from build123d import *

# Parameters (mm, degrees)
BOSS_EXTRUDE1_DEPTH        = 120
BOSS_EXTRUDE2_DEPTH        = 20
CUT_EXTRUDE1_DEPTH         = 20
SKETCH17_W                 = 82.2
SKETCH17_H                 = 120
BOSS_EXTRUDE3_DEPTH        = 20
SKETCH18_W                 = 15.5
SKETCH18_H                 = 23
CUT_EXTRUDE2_DEPTH         = 20
SKETCH19_W                 = 15.5
SKETCH19_H                 = 23
BOSS_EXTRUDE4_DEPTH        = 20
CUT_EXTRUDE3_DEPTH         = 37
FILLET3_R                  = 3
SKETCH22_W                 = 30
SKETCH22_H                 = 120
BOSS_EXTRUDE5_DEPTH        = 5
SKETCH23_W                 = 30
SKETCH23_H                 = 120
BOSS_EXTRUDE6_DEPTH        = 5
F_8_CLEARANCE_HOLE1_REACH  = 187.624
F_8_CLEARANCE_HOLE1_BORE_R = 2.2479


with BuildPart() as part:
    # Sketch1 → Boss-Extrude1 (new body)
    with BuildSketch(Plane(origin=(0, 0, 0), x_dir=(1, 0, 0), z_dir=(0, 1, 0))):
        Polygon((-70, 15), (-70, -15), (70, -15), (70, 15), (60.3, 15), (60.3, -5), (50.8, -5), (50.8, 15), (41.1, 15), (41.1, -5), (-41.1, -5), (-41.1, 15), (-50.8, 15), (-50.8, -5), (-60.3, -5), (-60.3, 15), align=None)
    extrude(amount=BOSS_EXTRUDE1_DEPTH)

    # Sketch2 → Boss-Extrude2 (add)
    with BuildSketch(Plane(origin=(0, 120, 0), x_dir=(1, 0, 0), z_dir=(0, 1, 0))):
        Polygon((-63.3, -8), (-63.3, 15), (-60.3, 15), (-60.3, -5), (-50.8, -5), (-50.8, 15), (-47.8, 15), (-47.8, -8), align=None)
        Polygon((63.3, -8), (63.3, 15), (60.3, 15), (60.3, -5), (50.8, -5), (50.8, 15), (47.8, 15), (47.8, -8), align=None)
    extrude(amount=BOSS_EXTRUDE2_DEPTH)

    # Sketch3 → Cut-Extrude1 (cut)
    with BuildSketch(Plane.XZ):
        Polygon((-47.8, 8), (-47.8, -15), (-50.8, -15), (-50.8, 5), (-60.3, 5), (-60.3, -15), (-63.3, -15), (-63.3, 8), align=None)
        Polygon((63.3, 8), (63.3, -15), (60.3, -15), (60.3, 5), (50.8, 5), (50.8, -15), (47.8, -15), (47.8, 8), align=None)
    extrude(amount=-CUT_EXTRUDE1_DEPTH, mode=Mode.SUBTRACT)

    # Sketch17 → Boss-Extrude3 (add)
    with BuildSketch(Plane(origin=(0, 0, 5), x_dir=(-1, 0, 0), z_dir=(0, 0, -1))):
        with Locations((0, 60)):
            Rectangle(SKETCH17_W, SKETCH17_H)
    extrude(amount=BOSS_EXTRUDE3_DEPTH)

    # Sketch18 → Cut-Extrude2 (cut)
    with BuildSketch(Plane.XZ):
        with Locations((-25.05, -3.5)):
            Rectangle(SKETCH18_W, SKETCH18_H)
        with Locations((25.05, -3.5)):
            Rectangle(SKETCH18_W, SKETCH18_H)
    extrude(amount=-CUT_EXTRUDE2_DEPTH, mode=Mode.SUBTRACT)

    # Sketch19 → Boss-Extrude4 (add)
    with BuildSketch(Plane(origin=(0, 120, 0), x_dir=(1, 0, 0), z_dir=(0, 1, 0))):
        with Locations((-25.05, 3.5)):
            Rectangle(SKETCH19_W, SKETCH19_H)
        with Locations((25.05, 3.5)):
            Rectangle(SKETCH19_W, SKETCH19_H)
    extrude(amount=BOSS_EXTRUDE4_DEPTH)

    # Sketch20 → Cut-Extrude3 (cut)
    with BuildSketch(Plane(origin=(0, 0, -15), x_dir=(-1, 0, 0), z_dir=(0, 0, -1))):
        Polygon((0, 25), (31.464278342, 25), (0, 55.968777895), (-31.464278342, 25), align=None)
        Polygon((45.8, 70), (45.8, 101.047518053), (14.255721658, 70), (45.8, 38.952481947), align=None)
        Polygon((0, 115), (-31.464278342, 115), (0, 84.031222105), (31.464278342, 115), align=None)
        Polygon((-45.8, 70), (-45.8, 101.047518053), (-14.255721658, 70), (-45.8, 38.952481947), align=None)
    extrude(amount=-CUT_EXTRUDE3_DEPTH, mode=Mode.SUBTRACT)

    # Fillet3
    fillet3_edges = [part.edges().sort_by_distance(p)[0] for p in [
        (-31.464278342, 115, 0),
        (0, 84.031222105, 0),
        (31.464278342, 115, 0),
        (-45.8, 38.952481947, 0),
        (-14.255721658, 70, 0),
        (-45.8, 101.047518053, 0),
        (45.8, 38.952481947, 0),
        (45.8, 101.047518053, 0),
        (14.255721658, 70, 0),
        (31.464278342, 25, 0),
        (0, 55.968777895, 0),
        (-31.464278342, 25, 0),
    ]]
    fillet(fillet3_edges, radius=FILLET3_R)

    # Sketch22 → Boss-Extrude5 (add)
    with BuildSketch(Plane(origin=(70, 0, 0), x_dir=(0, 0, -1), z_dir=(1, 0, 0))):
        with Locations((0, 60)):
            Rectangle(SKETCH22_W, SKETCH22_H)
    extrude(amount=BOSS_EXTRUDE5_DEPTH)

    # Sketch23 → Boss-Extrude6 (add)
    with BuildSketch(Plane.ZY.offset(70)):
        with Locations((0, 60)):
            Rectangle(SKETCH23_W, SKETCH23_H)
    extrude(amount=BOSS_EXTRUDE6_DEPTH)

    # #8 Clearance Hole1 bore (on position points) → #8 Clearance Hole1 (cut, up to next)
    with BuildSketch(Plane(origin=(-75, 107.5, -5), x_dir=(0, 0, -1), z_dir=(-1, 0, 0)), mode=Mode.PRIVATE) as f_8_clearance_hole1_sk1:
        Circle(F_8_CLEARANCE_HOLE1_BORE_R)
    f_8_clearance_hole1_tool1 = extrude(f_8_clearance_hole1_sk1.sketch, amount=-F_8_CLEARANCE_HOLE1_REACH, mode=Mode.PRIVATE) & part.part
    # #8 Clearance Hole1 bore (on position points) → #8 Clearance Hole1 (cut, up to next)
    with BuildSketch(Plane(origin=(-75, 107.5, -5), x_dir=(0, 0, -1), z_dir=(-1, 0, 0)), mode=Mode.PRIVATE) as f_8_clearance_hole1_sk2:
        with Locations((0, 75)):
            Circle(F_8_CLEARANCE_HOLE1_BORE_R)
    f_8_clearance_hole1_tool2 = extrude(f_8_clearance_hole1_sk2.sketch, amount=-F_8_CLEARANCE_HOLE1_REACH, mode=Mode.PRIVATE) & part.part
    add(f_8_clearance_hole1_tool1.solids().sort_by_distance((-75, 107.5, -5))[0], mode=Mode.SUBTRACT)
    add(f_8_clearance_hole1_tool2.solids().sort_by_distance((-75, 32.5, -5))[0], mode=Mode.SUBTRACT)


solid = part.part
Can you work these out from the model? Positions are in its coordinate system, mm. A direction names the side the tool comes from. Give positions to 0.01 mm unless a question says otherwise; leave off trailing zeros. Loops run counter-clockwise (first coordinate to the right, second up) from the corner with the lowest first, then second, coordinate; pieces in that order, holes last. Notation, with made-up numbers: M -33.5,89 L -12.5,89 A25 ccw -12.5,109 Z; hole C 83,8.5 d10. An arc over 180 degrees is marked long. One line per item, written item: value. Start each with the question number.
1) I'm going to push flat-ended pins straight in: pin 1 (8 mm diameter, centred on x = -53, y = 6.5, fed in from -Z); pin 2 (6 mm diameter, centred on y = 130.5, z = -4.5, fed in from +X); pin 3 (6 mm diameter, centred on y = 132, z = -5.5, fed in from -X). Where does each tip first touch, or does it pass through?
2) On a 3-axis mill with a long thin cutter (end or side, diameter ignored), from which of +Z, -Z, +X, -X, +Y, -Y can I reach the whole of each face in a straight line? I mean faces 1 (the face through (-32.8, 130, -3)), 2 (the face through (32.8, 10, -4)), 3 (the face through (-43.913, 43.329, 0.21)), 4 (the face through (60.3, 79, -5)). Say none if no direction works.
3) Thinking about a two-plate mould opening in Y: for faces 5 (the face through (-45.8, 70, 0)), 6 (the face through (0, 25, 0)), 7 (the face through (47.8, 10, -4)), 8 (the face through (25, 20, -3)), which applies, +Y half, -Y half, draft (parallel to the pull), parting line (faces both ways), or undercut?
4) If we section it at D-D, the plane y = 48.5: Write out the boundary of the cut face in (x, z).
5) If I drill on line 1 (Y direction, x = -71, z = -5); line 2 (Y direction, x = 10, z = 1); line 3 (X direction, y = 16.5, z = -7.5), over which ranges is the centre line in solid material (lowest first)? Write a range as [from, to].
6) If we section it at A-A, the plane z = 10.5: Write out the boundary of the cut face in (x, y), and give its area (3 significant figures).
7) If we section it at C-C, the plane x = -10: Write out the boundary of the cut face in (y, z), and give its area (3 significant figures).
8) If we section it at B-B, the plane z = -5: Give the number of separate pieces and of enclosed holes in the cut face, and give its area (3 significant figures).
Completed:
1. pin 1: stops at z = 8
1. pin 2: stops at x = 63.3
1. pin 3: stops at x = -63.3
2. face 1: +Z, -Z, +Y
2. face 2: -Z, -Y
2. face 3: +Z, -Z
2. face 4: -Z, +Y, -Y
3. face 5: undercut
3. face 6: undercut
3. face 7: draft
3. face 8: -Y half
4. outline: M -75,-15 L -60.3,-15 L -60.3,5 L -50.8,5 L -50.8,-15 L -45.8,-15 L -45.8,15 L -75,15 Z; M -36.1,-15 L -7.59,-15 L -7.59,15 L -36.1,15 Z; M 7.59,-15 L 36.1,-15 L 36.1,15 L 7.59,15 Z; M 45.8,-15 L 50.8,-15 L 50.8,5 L 60.3,5 L 60.3,-15 L 75,-15 L 75,15 L 45.8,15 Z
5. line 1: y = [0, 30.25], [34.75, 105.25], [109.75, 120]
5. line 2: y = [0, 25], [46.13, 93.87], [115, 120]
5. line 3: x = [-75, -63.3], [-47.8, -32.8], [-17.3, 17.3], [32.8, 47.8], [63.3, 75]
6. outline: M -75,0 L 75,0 L 75,120 L -75,120 Z; hole M -45.8,46.11 A3 ccw -40.7,43.98 L -16.43,67.86 A3 ccw -16.43,72.14 L -40.7,96.02 A3 ccw -45.8,93.89 Z; hole M -26.24,30.14 A3 ccw -24.14,25 L 24.14,25 A3 ccw 26.24,30.14 L 2.1,53.9 A3 ccw -2.1,53.9 Z; hole M -26.24,109.86 L -2.1,86.1 A3 ccw 2.1,86.1 L 26.24,109.86 A3 ccw 24.14,115 L -24.14,115 A3 ccw Z; hole M 16.43,67.86 L 40.7,43.98 A3 ccw 45.8,46.11 L 45.8,93.89 A3 ccw 40.7,96.02 L 16.43,72.14 A3 ccw Z
6. area: 14,200 mm^2
7. outline: M 0,-15 L 25,-15 L 25,15 L 0,15 Z; M 46.13,-15 L 93.87,-15 L 93.87,15 L 46.13,15 Z; M 115,-15 L 120,-15 L 120,15 L 115,15 Z
7. area: 2,330 mm^2
8. separate pieces: 5
8. enclosed holes: 4
8. area: 11,800 mm^2
